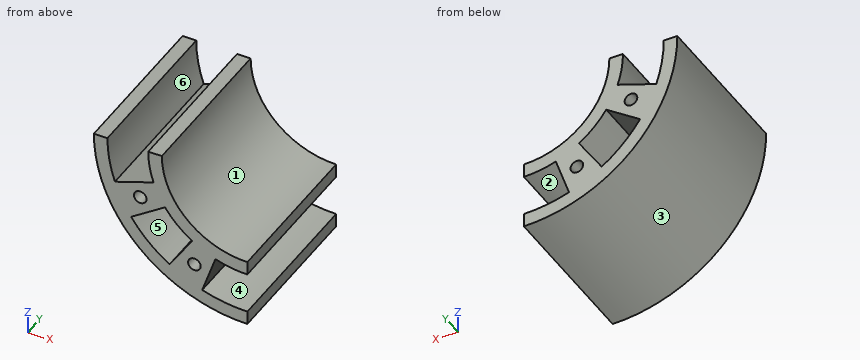
from build123d import *

# Parameters (mm, degrees)
SKETCH2_R           = 1.825
BOSS_EXTRUDE2_DEPTH = 46.8


with BuildPart() as part:
    # Sketch2 → Boss-Extrude2 (new body)
    with BuildSketch(Plane(origin=(0, 0, 0), x_dir=(1, 0, 0), z_dir=(0, 1, 0))):
        with BuildLine():
            Line((31.4, -60), (35.32, -60))
            ThreePointArc((35.32, -60), (42.54860464, -42.54860464), (60, -35.32))
            Line((60, -35.32), (60, -31.4))
            ThreePointArc((60, -31.4), (55.324247919, -31.784802987), (50.774317053, -32.928857169))
            Line((50.774317053, -32.928857169), (46.974367923, -21.778575262))
            ThreePointArc((46.974367923, -21.778575262), (53.398361223, -20.163298763), (60, -19.62))
            Line((60, -19.62), (60, -15.7))
            ThreePointArc((60, -15.7), (28.675169593, -28.675169593), (15.7, -60))
            Line((15.7, -60), (19.62, -60))
            ThreePointArc((19.62, -60), (20.163298763, -53.398361223), (21.778575262, -46.974367923))
            Line((21.778575262, -46.974367923), (32.928857169, -50.774317053))
            ThreePointArc((32.928857169, -50.774317053), (31.784802987, -55.324247919), (31.4, -60))
        make_face()
        with BuildLine():
            Line((37.529399815, -26.449790949), (44.084716065, -36.237345744))
            ThreePointArc((44.084716065, -36.237345744), (39.776746058, -39.776746058), (36.237345744, -44.084716065))
            Line((36.237345744, -44.084716065), (26.449790949, -37.529399815))
            ThreePointArc((26.449790949, -37.529399815), (31.447028176, -31.447028176), (37.529399815, -26.449790949))
        make_face(mode=Mode.SUBTRACT)
        with Locations((29.084372884, -44.71)):
            Circle(SKETCH2_R, mode=Mode.SUBTRACT)
        with Locations((44.71, -29.084372884)):
            Circle(SKETCH2_R, mode=Mode.SUBTRACT)
    extrude(amount=BOSS_EXTRUDE2_DEPTH)


solid = part.part
Geometry check sheet. Reference: the model listing, model coordinates, mm. Face numbers are marked on the shaded views. A direction names the side the tool comes from. Give positions to 0.01 mm unless a question says otherwise; leave off trailing zeros. Order: outer loops, then holes, each group sorted by start corner. A loop starts at its lowest first (then second) coordinate and runs counter-clockwise, first axis right, second up. Notation, with made-up numbers: (-24.5, 75) - (6.5, 75) arc R27 ccw to (6.5, 107) - close; hole circle Ø8 at (-39, 60). An arc over 180 degrees is marked (long way). Answer as a JSON object with one key per item and string values.
(1) Cross-section at C-C (y = 12.5). Record the cut outline in (x, z) (3 decimals), then the cut area to 3 significant figures.
Report:
{"outline": "(15.7, 60) arc R44.3 ccw to (60, 15.7) - (60, 19.62) arc R40.38 cw to (46.974, 21.779) - (50.774, 32.929) arc R28.6 ccw to (60, 31.4) - (60, 35.32) arc R24.68 cw to (35.32, 60) - (31.4, 60) arc R28.6 ccw to (32.929, 50.774) - (21.779, 46.974) arc R40.38 cw to (19.62, 60) - close; hole (26.45, 37.529) arc R40.38 ccw to (37.529, 26.45) - (44.085, 36.237) arc R28.6 cw to (36.237, 44.085) - close; hole circle Ø3.65 at (29.084, 44.71); hole circle Ø3.65 at (44.71, 29.084)", "area": "616 mm^2"}
(2) Tool access check on the marked faces 4, 5 and 6. Record the directions out of +Z, -Z, +X, -X, +Y, -Y that give a thin tool (end or side, any length) a straight path to the whole face; none if there is none.
Report:
{"face 4": "+X, +Y, -Y", "face 5": "+Y, -Y", "face 6": "+Z, +Y, -Y"}
(3) Cross-section at B-B (x = 57). Record the cut outline in (y, z), then the cut area to 3 significant figures.
Report:
{"outline": "(0, 15.8) - (46.8, 15.8) - (46.8, 19.73) - (0, 19.73) - close; (0, 31.56) - (46.8, 31.56) - (46.8, 35.5) - (0, 35.5) - close", "area": "369 mm^2"}
(4) Cross-section at A-A (z = 41.5). Record the cut outline in (x, y).
Report:
{"outline": "(19.75, 0) - (32.38, 0) - (32.38, 46.8) - (19.75, 46.8) - close; (38.19, 0) - (43.66, 0) - (43.66, 46.8) - (38.19, 46.8) - close"}
(5) Material ranges on line 1 (Z direction, x = 29, y = 30); line 2 (Z direction, x = 44, y = 17); line 3 (X direction, y = 34, z = 56.5), recorded low to high.
Report:
{"line 1": "28.35 to 34.12, 39.24 to 42.89, 46.53 to 49.44", "line 2": "18.69 to 27.4, 30.77 to 36.11, 36.29 to 41.21", "line 3": "15.84 to 19.77, 31.61 to 35.57"}
(6) Depth check by flat-ended pin: pin 1 Ø6 at (y, z) = (29, 41.5) entering from +X; pin 2 Ø6 at (x, y) = (48, 39.5) entering from -Z. Enter the tip coordinate at first touch or a pass-through.
Report:
{"pin 1": "x = 47.88", "pin 2": "z = 16.62"}
(7) Draft check along Z on the marked faces 1, 2 and 3. Enter one of: released by +Z, released by -Z, zero draft, split by the parting line, or undercut.
Report:
{"face 1": "released by +Z", "face 2": "undercut", "face 3": "released by -Z"}
